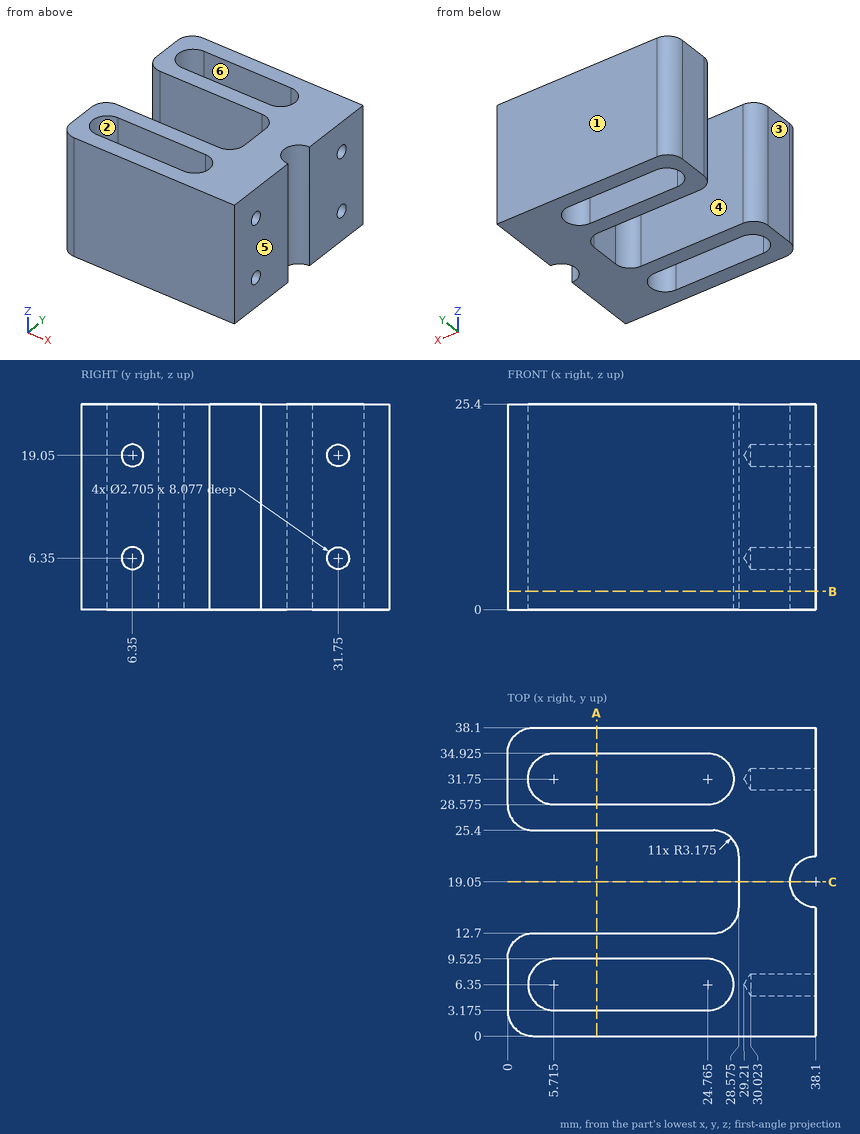
For this review, use the dimensioned drawing (mm, ordinates from the lowest corner) and the shaded views. A direction names the side the tool comes from. Round coordinates to 2 decimals unless told otherwise and drop trailing zeros. Loops run counter-clockwise (first coordinate to the right, second up) from the corner with the lowest first, then second, coordinate; pieces in that order, holes last. Notation, with made-up numbers: M 75,-11.75 L 125,-11.75 A21 ccw 125,14.25 Z; hole C 26,23.25 d3. An arc over 180 degrees is marked long. Answer as a JSON object with one key per item and string values.
(1) Tool access review of the marked faces 4, 5 and 6: name each direction out of +Z, -Z, +X, -X, +Y, -Y from which nothing blocks a thin tool from reaching the whole face with its end or side.
Resolved:
{"face 4": "+Z, -Z, -X", "face 5": "+Z, -Z, +X, +Y, -Y", "face 6": "+Z, -Z"}
(2) Take a section at A-A on x = 11. Give the boundary of the cut face in (y, z) (1 decimal).
Resolved:
{"outline": "M 0,0 L 3.2,0 L 3.2,25.4 L 0,25.4 Z; M 9.5,0 L 12.7,0 L 12.7,25.4 L 9.5,25.4 Z; M 25.4,0 L 28.6,0 L 28.6,25.4 L 25.4,25.4 Z; M 34.9,0 L 38.1,0 L 38.1,25.4 L 34.9,25.4 Z"}
(3) To check wall thickness, follow line 1 along Y through (x, z) = (21.5, 11.5) (1 decimal); line 2 along Y through (x, z) = (4, 13.5); line 3 along Z through (x, y) = (33, 6). State the ranges of each line that lie inside material, in increasing order.
Resolved:
{"line 1": "0 to 3.2, 9.5 to 12.7, 25.4 to 28.6, 34.9 to 38.1", "line 2": "0 to 3.68, 9.02 to 12.7, 25.4 to 29.08, 34.42 to 38.1", "line 3": "0 to 5.04, 7.66 to 17.74, 20.36 to 25.4"}
(4) Take a section at B-B on z = 2.25. Count the separate pieces of the cut face and the enclosed holes in it, and give its area (3 significant figures).
Resolved:
{"separate pieces": "1", "enclosed holes": "2", "area": "763 mm²"}
(5) Clearance check with flat-ended pins moving along their axes: P1, Ø1.6, axis at y = 6.35, z = 6.35, coming from the +X side; P2, Ø5, axis at y = 17.5, z = 17.5, coming from the -X side; P3, Ø2, axis at y = 31.75, z = 19.05, coming from the +X side. State where each tip first meets the part, or that it passes through.
Resolved:
{"P1": "x = 29.69", "P2": "x = 28.45", "P3": "x = 29.81"}
(6) Take a section at C-C on y = 19.05. Give the boundary of the cut face in (x, z) (1 decimal), and give its area (3 significant figures).
Resolved:
{"outline": "M 28.6,0 L 34.9,0 L 34.9,25.4 L 28.6,25.4 Z", "area": "161 mm²"}
(7) Draft analysis for pull direction Y (two halves, no side actions). For the marked faces 1, 2 and 3, state which applies: released by +Y, released by -Y, zero draft, split by the parting line, or undercut.
Resolved:
{"face 1": "released by +Y", "face 2": "undercut", "face 3": "zero draft"}
